Source: CAD feature listing. Evaluate the final solid. Frame: model axes, mm. A direction names the side the tool comes from. Coordinates: 2 decimals unless noted, no trailing zeros. Loops run counter-clockwise (first coordinate to the right, second up) from the corner with the lowest first, then second, coordinate; pieces in that order, holes last.
from build123d import *

# Parameters (mm, degrees)
F0_R     = 4.445
F0_R_2   = 3.175
F1_DEPTH = 3.175
F2_R     = 4.064
F2_R_2   = 3.429
F3_DEPTH = 1.27
F4_R     = 1.016
F5_W     = 6.35
F5_H     = 3.175
F6_DEPTH = 25.4


with BuildPart() as f1:
    # F0 (on Top) → F1 (new body)
    with BuildSketch(Plane.XY):
        Circle(F0_R)
        Circle(F0_R_2, mode=Mode.SUBTRACT)
    extrude(amount=F1_DEPTH)

    # F2 (on face) → F3 (cut)
    with BuildSketch(Plane.XY.offset(3.175)):
        Circle(F2_R)
        Circle(F2_R_2, mode=Mode.SUBTRACT)
    extrude(amount=-F3_DEPTH, mode=Mode.SUBTRACT)

    # F4
    f4_edges = [f1.edges().sort_by_distance(p)[0] for p in [
        (-3.175, 0, 0),
    ]]
    fillet(f4_edges, radius=F4_R)

    # F5 (on Top) → F6 (cut)
    with BuildSketch(Plane.XY):
        with Locations((-3.175, 0)):
            Rectangle(F5_W, F5_H)
    extrude(amount=F6_DEPTH, mode=Mode.SUBTRACT)


solid = f1.part
Q1. Line query: line 1 along X through (y, z) = (-2.25, 2.25); line 2 along X through (y, z) = (-1.75, 1.6); line 3 along Y through (x, z) = (-3.5, 1.6). Output: solid intervals per line, ascending.
Q2. Section A-A, the plane x = 0. Return the cut outline in (y, z) (3 decimals).
Q3. Draft query along X for faces 4 (the flat face through (3, -2, 1.905)), 5 (the cylindrical face through (4.44, -0.17, 1.57)), 6 (the flat face through (-3.5, 1.588, 1.6)). Return one class per face: +X half, -X half, draft (parallel to the pull), parting line (faces both ways), or undercut.
Q4. Contact query for flat-ended pins moving along their axis: pin 1 Ø1 at (x, y) = (2, -2.5) entering from -Z; pin 2 Ø5 at (x, y) = (0, 0) entering from -Z; pin 3 Ø0.7 at (x, z) = (-3, 2.5) entering from +Y. Output: stop coordinate, or through.
Q5. Access query for faces 1 (the flat face through (-3.5, -1.588, 1.6)), 2 (the flat face through (4.27, 0.02, 3.175)), 3 (the cylindrical face through (4.06, -0.16, 2.55)). Directions: +Z, -Z, +X, -X, +Y, -Y. A direction counts if a zero-diameter tool reaches every point of the face in a straight line with its end or side. Return the directions, or none.
Q6. Section C-C, the plane y = 0. Return the cut outline in (x, z) (3 decimals), plus the area to 3 significant figures.
Derived:
1. line 1: x = -3.83 to -3.38, -2.59 to -2.24, 2.24 to 2.59, 3.38 to 3.83
1. line 2: x = -4.09 to -2.65, 2.65 to 4.09
1. line 3: y = -2.74 to -1.59, 1.59 to 2.74
2. outline: (-4.445, 0) - (-4.191, 0) arc R1.016 ccw to (-3.175, 1.016) - (-3.175, 3.175) - (-3.429, 3.175) - (-3.429, 1.905) - (-4.064, 1.905) - (-4.064, 3.175) - (-4.445, 3.175) - close; (3.175, 1.016) arc R1.016 ccw to (4.191, 0) - (4.445, 0) - (4.445, 3.175) - (4.064, 3.175) - (4.064, 1.905) - (3.429, 1.905) - (3.429, 3.175) - (3.175, 3.175) - close
3. face 4: undercut
3. face 5: parting line
3. face 6: draft
4. pin 1: stops at z = 0.13
4. pin 2: passes through
4. pin 3: stops at y = 3.57
5. face 1: +Z, -Z, -X
5. face 2: +Z, +X, -X, +Y, -Y
5. face 3: +Z
6. outline: (3.175, 1.016) arc R1.016 ccw to (4.191, 0) - (4.445, 0) - (4.445, 3.175) - (4.064, 3.175) - (4.064, 1.905) - (3.429, 1.905) - (3.429, 3.175) - (3.175, 3.175) - close
6. area: 3.00 mm2
